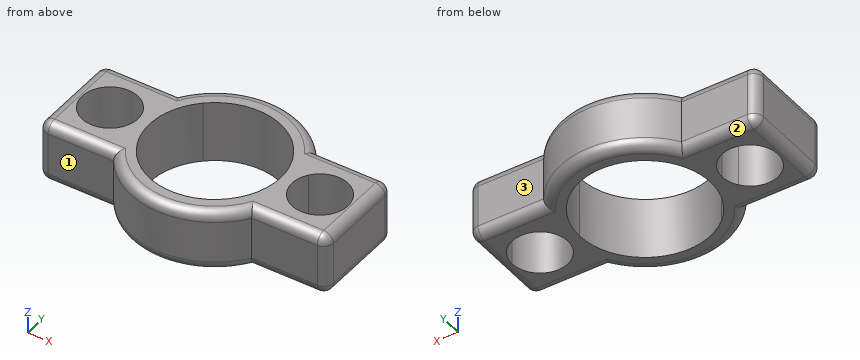
from build123d import *

# Parameters (mm, degrees)
F1_DEPTH = 12.7
F2_R     = 2


with BuildPart() as f1:
    # F0 (on Top) → F1 (new body)
    with BuildSketch(Plane.XY):
        with BuildLine():
            ThreePointArc((-17.164541762, -3.4100595449), (-16.1036698951, -6.8499500663), (-14.3614066163, -10))
            Line((-14.3614066163, -10), (-9.2173748974, -10))
            ThreePointArc((-9.2173748974, -10), (-13.6, 0), (-9.2173748974, 10))
            Line((-9.2173748974, 10), (-14.3614066163, 10))
            ThreePointArc((-14.3614066163, 10), (-16.1036698951, 6.8499500663), (-17.164541762, 3.4100595449))
            ThreePointArc((-17.164541762, 3.4100595449), (-16.3393623105, 1.7930134566), (-16.055, 0))
            ThreePointArc((-16.055, 0), (-16.3393623105, -1.7930134566), (-17.164541762, -3.4100595449))
        make_face()
        with BuildLine():
            Line((9.2173748974, 10), (14.3614066163, 10))
            ThreePointArc((14.3614066163, 10), (0, 17.5), (-14.3614066163, 10))
            Line((-14.3614066163, 10), (-9.2173748974, 10))
            ThreePointArc((-9.2173748974, 10), (0, 13.6), (9.2173748974, 10))
        make_face()
        with BuildLine():
            ThreePointArc((-14.3614066163, -10), (0, -17.5), (14.3614066163, -10))
            Line((14.3614066163, -10), (9.2173748974, -10))
            ThreePointArc((9.2173748974, -10), (0, -13.6), (-9.2173748974, -10))
            Line((-9.2173748974, -10), (-14.3614066163, -10))
        make_face()
        with BuildLine():
            Line((9.2173748974, -10), (14.3614066163, -10))
            ThreePointArc((14.3614066163, -10), (16.1036698951, -6.8499500663), (17.164541762, -3.4100595449))
            ThreePointArc((17.164541762, -3.4100595449), (16.055, 0), (17.164541762, 3.4100595449))
            ThreePointArc((17.164541762, 3.4100595449), (16.1036698951, 6.8499500663), (14.3614066163, 10))
            Line((14.3614066163, 10), (9.2173748974, 10))
            ThreePointArc((9.2173748974, 10), (12.4562494075, 5.4591071337), (13.6, 0))
            ThreePointArc((13.6, 0), (12.4562494075, -5.4591071337), (9.2173748974, -10))
        make_face()
        with BuildLine():
            Line((14.3614066163, -10), (30, -10))
            Line((30, -10), (30, 10))
            Line((30, 10), (14.3614066163, 10))
            ThreePointArc((14.3614066163, 10), (16.1036698951, 6.8499500663), (17.164541762, 3.4100595449))
            ThreePointArc((17.164541762, 3.4100595449), (23.6430134566, 5.5106376895), (27.645, 0))
            ThreePointArc((27.645, 0), (23.6430134566, -5.5106376895), (17.164541762, -3.4100595449))
            ThreePointArc((17.164541762, -3.4100595449), (16.1036698951, -6.8499500663), (14.3614066163, -10))
        make_face()
        with BuildLine():
            Line((-30, -10), (-14.3614066163, -10))
            ThreePointArc((-14.3614066163, -10), (-16.1036698951, -6.8499500663), (-17.164541762, -3.4100595449))
            ThreePointArc((-17.164541762, -3.4100595449), (-27.645, 0), (-17.164541762, 3.4100595449))
            ThreePointArc((-17.164541762, 3.4100595449), (-16.1036698951, 6.8499500663), (-14.3614066163, 10))
            Line((-14.3614066163, 10), (-30, 10))
            Line((-30, 10), (-30, -10))
        make_face()
    extrude(amount=F1_DEPTH)

    # F2
    f2_edges = [f1.edges().sort_by_distance(p)[0] for p in [
        (-22.180703, -10, 12.7),
        (0, -17.5, 12.7),
        (22.180703, -10, 12.7),
        (30, 0, 12.7),
        (-30, 0, 12.7),
        (-22.180703, 10, 12.7),
        (0, 17.5, 12.7),
        (22.180703, 10, 12.7),
        (30, 10, 6.35),
        (-30, 10, 6.35),
        (-30, -10, 6.35),
        (30, -10, 6.35),
        (0, -17.5, 0),
        (-22.180703, -10, 0),
        (-30, 0, 0),
        (-22.180703, 10, 0),
        (0, 17.5, 0),
        (22.180703, 10, 0),
        (30, 0, 0),
        (22.180703, -10, 0),
    ]]
    fillet(f2_edges, radius=F2_R)


solid = f1.part
Read the model definition and answer for the solid it produces. Units are mm, in the model's axes. Face numbers are marked on the shaded views. A direction names the side the tool comes from. Round coordinates to 2 decimals unless told otherwise and drop trailing zeros. Order: outer loops, then holes, each group sorted by start corner. A loop starts at its lowest first (then second) coordinate and runs counter-clockwise, first axis right, second up.
1) For the marked faces 1, 2 and 3, determine the directions among +Z, -Z, +X, -X, +Y, -Y from which every point of the face is accessible in a straight line to the end or side of a thin tool.
2) Flat-ended cylindrical pins translate along their axes: pin 1 (2.5 mm diameter, centred on x = 21.5, z = 7, fed in from +Y); pin 2 (4.5 mm diameter, centred on x = 23.5, z = 8, fed in from -Y); pin 3 (9.5 mm diameter, centred on x = -21.85, y = 0, fed in from +Z); pin 4 (3 mm diameter, centred on x = 9.5, z = 2, fed in from -Y). Find the tip coordinate at first contact, or state that the pin passes through.
3) The part is cut by section A-A on x = 0. Write down the section's boundary in (y, z).
4) The part is cut by section C-C on y = 2. Write down the section's boundary in (x, z), plus the area to 3 significant figures.
5) The part is cut by section B-B on z = 9. Write down the section's boundary in (x, y) (3 decimals).
6) The part is cut by section D-D on x = -21.85. Write down the section's boundary in (y, z) (3 decimals), plus the area to 3 significant figures.
7) Straight lines are drawn through the part: L1, parallel to Y at x = -21.85, z = 8.5 (3 decimals); L2, parallel to X at y = -11, z = 5.5; L3, parallel to Y at x = -0.5, z = 8. For each, find the intervals that lie inside material, in ascending order.
Resolved:
1. face 1: +Z, -Z, -X, -Y
1. face 2: -Z, -X, +Y
1. face 3: +Z, -Z, +X, +Y
2. pin 1: stops at y = 10
2. pin 2: stops at y = -10
2. pin 3: passes through
2. pin 4: stops at y = -15.56
3. outline: (-17.5, 2) arc R2 ccw to (-15.5, 0) - (-13.6, 0) - (-13.6, 12.7) - (-15.5, 12.7) arc R2 ccw to (-17.5, 10.7) - close; (13.6, 0) - (15.5, 0) arc R2 ccw to (17.5, 2) - (17.5, 10.7) arc R2 ccw to (15.5, 12.7) - (13.6, 12.7) - close
4. outline: (-30, 2) arc R2 ccw to (-28, 0) - (-27.29, 0) - (-27.29, 12.7) - (-28, 12.7) arc R2 ccw to (-30, 10.7) - close; (-16.41, 0) - (-13.45, 0) - (-13.45, 12.7) - (-16.41, 12.7) - close; (13.45, 0) - (16.41, 0) - (16.41, 12.7) - (13.45, 12.7) - close; (27.29, 0) - (28, 0) arc R2 ccw to (30, 2) - (30, 10.7) arc R2 ccw to (28, 12.7) - (27.29, 12.7) - close
4. area: 141 mm2
5. outline: (-30, -8) arc R2 ccw to (-28, -10) - (-14.361, -10) arc R17.5 ccw to (14.361, -10) - (28, -10) arc R2 ccw to (30, -8) - (30, 8) arc R2 ccw to (28, 10) - (14.361, 10) arc R17.5 ccw to (-14.361, 10) - (-28, 10) arc R2 ccw to (-30, 8) - close; hole circle Ø11.59 at (-21.85, 0); hole circle Ø27.2 at (0, 0); hole circle Ø11.59 at (21.85, 0)
6. outline: (-10, 2) arc R2 ccw to (-8, 0) - (-5.795, 0) - (-5.795, 12.7) - (-8, 12.7) arc R2 ccw to (-10, 10.7) - close; (5.795, 0) - (8, 0) arc R2 ccw to (10, 2) - (10, 10.7) arc R2 ccw to (8, 12.7) - (5.795, 12.7) - close
6. area: 103 mm2
7. L1: y = -10 to -5.795, 5.795 to 10
7. L2: x = -13.61 to -8, 8 to 13.61
7. L3: y = -17.49 to -13.59, 13.59 to 17.49
